For this review, take the finished solid that the model builds, in its own axes (mm). Face numbers are marked on the shaded views. A direction names the side the tool comes from. Coordinates: 2 decimals unless noted, no trailing zeros. Loops run counter-clockwise (first coordinate to the right, second up) from the corner with the lowest first, then second, coordinate; pieces in that order, holes last. Notation, with made-up numbers: (-24.5, 37) -> (-6.5, 37) arc R28 cw to (-6.5, 69) -> close; hole circle Ø4 at (25, 82.25). An arc over 180 degrees is marked (long way). Use a Markdown table: item, result.
from build123d import *

# Parameters (mm, degrees)
CROQUIS1_W              = 151.3
CROQUIS1_H              = 148
SALIENTE_EXTRUIR1_DEPTH = 1.8
CROQUIS2_W              = 151.3
CROQUIS2_H              = 148
CROQUIS2_W_2            = 147.1
CROQUIS2_H_2            = 143.8
SALIENTE_EXTRUIR2_DEPTH = 18.2
CROQUIS4_R              = 6.25
CROQUIS4_R_2            = 3.5
CROQUIS4_R_3            = 4
CORTAR_EXTRUIR1_DEPTH   = 2.1
CROQUIS5_R              = 1
SALIENTE_EXTRUIR3_DEPTH = 15.5


with BuildPart() as part:
    # Croquis1 → Saliente-Extruir1 (new body)
    with BuildSketch(Plane.XY):
        with Locations((-105.482201909, -12.901601831)):
            Rectangle(CROQUIS1_W, CROQUIS1_H)
    extrude(amount=SALIENTE_EXTRUIR1_DEPTH)

    # Croquis2 → Saliente-Extruir2 (add)
    with BuildSketch(Plane.XY.offset(1.8)):
        with Locations((-105.482201909, -12.901601831)):
            Rectangle(CROQUIS2_W, CROQUIS2_H)
        with Locations((-105.482201909, -12.901601831)):
            Rectangle(CROQUIS2_W_2, CROQUIS2_H_2, mode=Mode.SUBTRACT)
    extrude(amount=SALIENTE_EXTRUIR2_DEPTH)

    # Croquis4 → Cortar-Extruir1 (cut)
    with BuildSketch(Plane(origin=(0, 61.098398169, 0), x_dir=(1, 0, 0), z_dir=(0, 1, 0))):
        with Locations(Location((-104.482201909, -9.1, 0), (0, 0, 270))):
            Circle(CROQUIS4_R)
        with Locations(Location((-163.132201909, -6.3, 0), (0, 0, 270))):
            Circle(CROQUIS4_R_2)
        with Locations(Location((-133.132201909, -7.05, 0), (0, 0, 270))):
            Circle(CROQUIS4_R_3)
    extrude(amount=-CORTAR_EXTRUIR1_DEPTH, mode=Mode.SUBTRACT)

    # Croquis5 → Saliente-Extruir3 (add)
    with BuildSketch(Plane.XY.offset(1.8)):
        with BuildLine():
            Line((-133.94514144, -4.251601831), (-133.94514144, -6.651601831))
            Line((-133.94514144, -6.651601831), (-162.94514144, -6.651601831))
            Line((-162.94514144, -6.651601831), (-162.94514144, -19.151601831))
            Line((-162.94514144, -19.151601831), (-133.94514144, -19.151601831))
            Line((-133.94514144, -19.151601831), (-133.94514144, -21.551601831))
            Line((-133.94514144, -21.551601831), (-162.94514144, -21.551601831))
            ThreePointArc((-162.94514144, -21.551601831), (-168.04514144, -12.901601831), (-162.94514144, -4.251601831))
            Line((-162.94514144, -4.251601831), (-133.94514144, -4.251601831))
        make_face()
        with Locations((-165.49514144, -12.901601831)):
            Circle(CROQUIS5_R, mode=Mode.SUBTRACT)
    extrude(amount=SALIENTE_EXTRUIR3_DEPTH)


solid = part.part
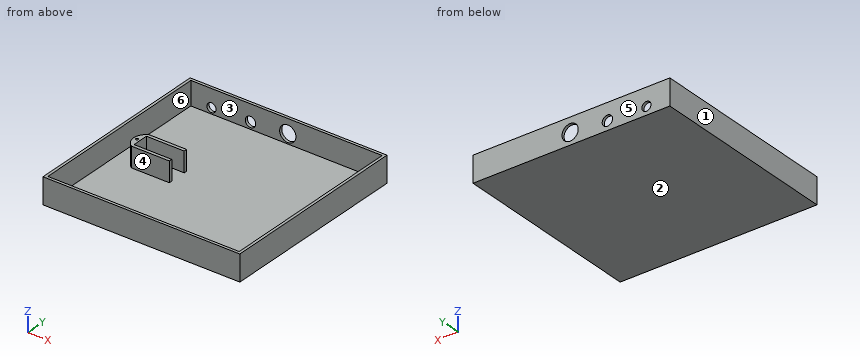
(1) Take a section at D-D on x = -131. Write out the cut boundary in (y, z).
Found:
| item | result |
|---|---|
| outline | (-86.9, 0) -> (61.1, 0) -> (61.1, 3.67) -> (59, 3.67) -> (59, 1.8) -> (-84.8, 1.8) -> (-84.8, 20) -> (-86.9, 20) -> close; (59, 10.43) -> (61.1, 10.43) -> (61.1, 20) -> (59, 20) -> close |
(2) Take a section at C-C on y = -66. Write out the cut boundary in (x, z), plus the area to 3 significant figures.
Found:
| item | result |
|---|---|
| outline | (-181.13, 0) -> (-29.83, 0) -> (-29.83, 20) -> (-31.93, 20) -> (-31.93, 1.8) -> (-179.03, 1.8) -> (-179.03, 20) -> (-181.13, 20) -> close |
| area | 349 mm^2 |
(3) For the marked faces 5 and 6, list the 3-axis set-ups (+Z, -Z, +X, -X, +Y, -Y) from which the entire face can be reached by the end or side of a thin tool; tool diameter is ignored.
Found:
| item | result |
|---|---|
| face 5 | +Z, -Z, +X, -X, +Y |
| face 6 | +Z |
(4) Take a section at B-B on x = -41. Write out the cut boundary in (y, z).
Found:
| item | result |
|---|---|
| outline | (-86.9, 0) -> (61.1, 0) -> (61.1, 20) -> (59, 20) -> (59, 1.8) -> (-84.8, 1.8) -> (-84.8, 20) -> (-86.9, 20) -> close |
(5) For line 1 along Y through (x, z) = (-154.5, 3.5); line 2 along X through (y, z) = (-42.5, 16.5); line 3 along Y through (x, z) = (-77, 3.25), list the stretches that pass through material, from the lowest coordinate up.
Found:
| item | result |
|---|---|
| line 1 | y = -86.9 to -84.8, -21.55 to -19.15, -6.65 to -4.25, 59 to 61.1 |
| line 2 | x = -181.13 to -179.03, -31.93 to -29.83 |
| line 3 | y = -86.9 to -84.8, 59 to 61.1 |
(6) For pin 1 Ø4 at (x, y) = (-67, -36.5) entering from +Z; pin 2 Ø2.5 at (x, y) = (-165.5, -12.9) entering from +Z; pin 3 Ø11 at (x, z) = (-104.48, 9.1) entering from +Y, all flat-tipped, find the tip position at first contact; note any pin that passes through.
Found:
| item | result |
|---|---|
| pin 1 | stops at z = 1.8 |
| pin 2 | stops at z = 17.3 |
| pin 3 | stops at y = -84.8 |
(7) Mouldability with a two-part tool opening along X and no side actions: class the marked faces 1, 2, 3 and 4 as pulls with the +X half, pulls with the -X half, needs draft (parallel to the pull), parting line crosses it, or undercut.
Found:
| item | result |
|---|---|
| face 1 | pulls with the -X half |
| face 2 | needs draft |
| face 3 | undercut |
| face 4 | undercut |
(8) Take a section at A-A on z = 7.05. State how many separate pieces and enclosed holes the cut face has, plus the area to 3 significant figures.
Found:
| item | result |
|---|---|
| separate pieces | 4 |
| enclosed holes | 1 |
| area | 1,380 mm^2 |
